```python
from build123d import *

# Parameters (mm, degrees)
BOSS_EXTRUDE1_DEPTH = 200
FILLET1_R           = 5
CHAMFER1_SIZE       = 18
SKETCH2_R           = 2.6
CUT_EXTRUDE1_DEPTH  = 207.968596652


with BuildPart() as part:
    # Sketch1 → Boss-Extrude1 (new body)
    with BuildSketch(Plane.XY):
        with BuildLine():
            Line((-20, 20), (-20, 30))
            Line((-20, 30), (-24, 30))
            Line((-24, 30), (-24, 4))
            Line((-24, 4), (-44, 4))
            Line((-44, 4), (-44, 0))
            Line((-44, 0), (-24, 0))
            Line((-24, 0), (-24, -20))
            Line((-24, -20), (-20, -20))
            Line((-20, -20), (-20, -4))
            Line((-20, -4), (20, -4))
            Line((20, -4), (20, -20))
            Line((20, -20), (24, -20))
            Line((24, -20), (24, 0))
            Line((24, 0), (44, 0))
            Line((44, 0), (44, 4))
            Line((44, 4), (24, 4))
            Line((24, 4), (24, 30))
            Line((24, 30), (20, 30))
            Line((20, 30), (20, 20))
            ThreePointArc((20, 20), (0, 0), (-20, 20))
        make_face()
    extrude(amount=BOSS_EXTRUDE1_DEPTH)

    # Fillet1
    fillet1_edges = [part.edges().sort_by_distance(p)[0] for p in [
        (24, 4, 100),
        (-24, 4, 100),
    ]]
    fillet(fillet1_edges, radius=FILLET1_R)

    # Chamfer1
    # the kernel refuses this chamfer: 18 mm, written as the material it adds along each edge
    with BuildSketch(Plane(origin=(20, -4, 0), x_dir=(-0.9996219169112966, 0.027495876610586365, 0), z_dir=(0, 0, 1))) as chamfer1_piece_1_section:
        Polygon((CHAMFER1_SIZE * 0.999621916911, CHAMFER1_SIZE * 0.0274958766106), (-CHAMFER1_SIZE * 0.0274958766106, CHAMFER1_SIZE * 0.999621916911), (0, 0), align=None)
    chamfer1_piece_1 = extrude(amount=200, mode=Mode.PRIVATE)
    chamfer1_piece_1 = split(chamfer1_piece_1, bisect_by=Plane(origin=(13.93765318, -20, 100), z_dir=(0, 1, 0)), keep=Keep.TOP, mode=Mode.PRIVATE)
    add(chamfer1_piece_1)
    with BuildSketch(Plane(origin=(-20, -4, 0), x_dir=(-0.027495876610586584, -0.9996219169112966, 0), z_dir=(0, 0, 1))) as chamfer1_piece_2_section:
        Polygon((CHAMFER1_SIZE * 0.999621916911, CHAMFER1_SIZE * 0.0274958766106), (-CHAMFER1_SIZE * 0.0274958766106, CHAMFER1_SIZE * 0.999621916911), (0, 0), align=None)
    chamfer1_piece_2 = extrude(amount=200, mode=Mode.PRIVATE)
    chamfer1_piece_2 = split(chamfer1_piece_2, bisect_by=Plane(origin=(-13.93765318, -20, 100), z_dir=(0, 1, 0)), keep=Keep.TOP, mode=Mode.PRIVATE)
    add(chamfer1_piece_2)

    # Sketch2 → Cut-Extrude1 (cut, through all)
    with BuildSketch(Plane.XZ):
        with Locations(Location((-34, 190, 0), (0, 0, 270))):
            Circle(SKETCH2_R)
        with Locations(Location((-34, 160, 0), (0, 0, 270))):
            Circle(SKETCH2_R)
        with Locations(Location((-34, 130, 0), (0, 0, 270))):
            Circle(SKETCH2_R)
        with Locations(Location((-34, 100, 0), (0, 0, 270))):
            Circle(SKETCH2_R)
        with Locations(Location((-34, 70, 0), (0, 0, 270))):
            Circle(SKETCH2_R)
        with Locations(Location((-34, 40, 0), (0, 0, 270))):
            Circle(SKETCH2_R)
        with Locations(Location((-34, 10, 0), (0, 0, 270))):
            Circle(SKETCH2_R)
        with Locations((34, 10)):
            Circle(SKETCH2_R)
        with Locations((34, 40)):
            Circle(SKETCH2_R)
        with Locations((34, 70)):
            Circle(SKETCH2_R)
        with Locations((34, 100)):
            Circle(SKETCH2_R)
        with Locations((34, 130)):
            Circle(SKETCH2_R)
        with Locations((34, 160)):
            Circle(SKETCH2_R)
        with Locations((34, 190)):
            Circle(SKETCH2_R)
    extrude(amount=-CUT_EXTRUDE1_DEPTH, mode=Mode.SUBTRACT)


solid = part.part
```
Input: part model. Units: mm. Frame: model coordinates. A direction names the side the tool comes from. Give positions to 0.01 mm unless a question says otherwise; leave off trailing zeros. Loops run counter-clockwise (first coordinate to the right, second up) from the corner with the lowest first, then second, coordinate; pieces in that order, holes last. Notation, with made-up numbers: (52, 72.5) -> (57, 72.5) arc R31 ccw to (57, 99.5) -> close; hole circle Ø10 at (74, 77). An arc over 180 degrees is marked (long way). Use a Markdown table: item, result.
Q1. Access query for faces 4 (the flat face through (-20, 25, 99)), 5 (the flat face through (-10, -12, 99)), 6 (the flat face through (-24, -10, 99)), 7 (the flat face through (37, 4, 99)). Directions: +Z, -Z, +X, -X, +Y, -Y. A direction counts if a zero-diameter tool reaches every point of the face in a straight line with its end or side. Return the directions, or none.
Entries:
| item | result |
|---|---|
| face 4 | +Z, -Z, +Y |
| face 5 | +Z, -Z, -Y |
| face 6 | +Z, -Z, -X, -Y |
| face 7 | +Z, -Z, +X, +Y |
Q2. Ray query, probe 1 along Y at (x, z) = (1, 181); probe 2 along X at (y, z) = (6, 145); probe 3 along Y at (x, z) = (28.5, 174.5). Return the intervals inside material, ascending. Write a range as from..to.
Entries:
| item | result |
|---|---|
| probe 1 | y = -4..0.03 |
| probe 2 | x = -25..-14.28, 14.28..25 |
| probe 3 | y = 0..4.03 |
Q3. Pull-direction query (X, two-part tool) for faces 1 (the flat face through (21, -20, 99)), 2 (the cylindrical face through (-33.9, 2, 42.6)), 3 (the flat face through (44, 2, 99)); classes: pulls with the +X half, pulls with the -X half, needs draft (parallel to the pull), parting line crosses it, or undercut.
Entries:
| item | result |
|---|---|
| face 1 | needs draft |
| face 2 | undercut |
| face 3 | pulls with the +X half |
Q4. Section query D-D, the plane x = -9. Return the cut outline in (y, z).
Entries:
| item | result |
|---|---|
| outline | (-11, 0) -> (2.14, 0) -> (2.14, 200) -> (-11, 200) -> close |
Q5. Section query C-C, the plane x = 0. Return the cut outline in (y, z).
Entries:
| item | result |
|---|---|
| outline | (-4, 0) -> (0, 0) -> (0, 200) -> (-4, 200) -> close |
Q6. First-contact query: P1, Ø1.2, axis at x = -0.5, z = 131.5, coming from the -Y side; P2, Ø22, axis at x = -37, z = 111, coming from the -Y side; P3, Ø4, axis at y = 14.5, z = 94, coming from the +X side; P4, Ø8, axis at x = 15.5, y = 17.5, coming from the +Z side. Flat tips, straight axial feed; report the tip coordinate or a pass-through.
Entries:
| item | result |
|---|---|
| P1 | stops at y = -4 |
| P2 | stops at y = 0 |
| P3 | stops at x = 24 |
| P4 | passes through |
Q7. Section query A-A, the plane x = 34. State how many separate pieces and enclosed holes the cut face has, plus the area to 3 significant figures.
Entries:
| item | result |
|---|---|
| separate pieces | 8 |
| enclosed holes | 0 |
| area | 654 mm² |
